```python
from build123d import *

# Parameters (mm, degrees)
F0_W     = 134.62
F0_H     = 76.2
F1_DEPTH = 15.875
F3_DEPTH = 76.201
F5_DEPTH = 83.5152


with BuildPart() as f1:
    # F0 (on Top) → F1 (new body, symmetric)
    with BuildSketch(Plane.XY):
        Rectangle(F0_W, F0_H)
    extrude(amount=F1_DEPTH, both=True)

    # F2 (on face) → F3 (cut, through all)
    with BuildSketch(Plane.XZ.offset(38.1)):
        Polygon((-33.401, 15.875), (-49.911, 15.875), (-49.911, 0), (-54.6735, 0), (-54.6735, -8.255), (-28.6385, -8.255), (-28.6385, 0), (-33.401, 0), align=None)
    extrude(amount=-F3_DEPTH, mode=Mode.SUBTRACT)

    # F4 (on face) → F5 (cut)
    with BuildSketch(Plane.YZ.offset(67.31)):
        with BuildLine():
            ThreePointArc((13.990774, -8.396005), (0.020774, 5.573995), (-13.949226, -8.396005))
            Line((-13.949226, -8.396005), (13.990774, -8.396005))
        make_face()
        Polygon((-13.949226, -8.396005), (-22.204226, -8.396005), (-17.886226, -15.875), (17.927774, -15.875), (22.245774, -8.396005), (13.990774, -8.396005), align=None)
    extrude(amount=-F5_DEPTH, mode=Mode.SUBTRACT)


with BuildPart() as f6_1:
    # F6: copy of F1
    add(f1.part)


solid = f1.part
```
Part model, mm, in its own coordinate system. A direction names the side the tool comes from. Give positions to 0.01 mm unless a question says otherwise; leave off trailing zeros. Order: outer loops, then holes, each group sorted by start corner. A loop starts at its lowest first (then second) coordinate and runs counter-clockwise, first axis right, second up. Notation, with made-up numbers: M 20,55 L 59,55 A30 cw 59,94 Z; hole C 27.25,6.5 d9. An arc over 180 degrees is marked long. Use a Markdown table: item, result. Add a question column.
(1) Drop flat-ended pins along their axis: P1, Ø9, axis at y = -5, z = -3.5, coming from the +X side; P2, Ø8, axis at x = -40, y = -17, coming from the +Z side (3 decimals). Give the stop position or say it passes through.
(2) Saw through at C-C, the plane x = -3.5. Give the cut face in (y, z) (3 decimals), and give its area (3 significant figures).
(3) Mould opens along Z. For faces 4 (the face through (26.14, 0.33, 5.57)), 5 (the face through (-59, 1, 15.875)), 6 (the face through (26.137, -20.075, -12.083)) say: +Z half, -Z half, draft (parallel to the pull), parting line (faces both ways), or undercut.
(4) Saw through at A-A, the plane z = -5. Give the cut face in (x, y).
(5) 3-axis set-ups, long thin cutter, end or side, ignore diameter. For faces 1 (the face through (-49.911, -1, 8)), 2 (the face through (26, -18, -8.396)), 3 (the face through (-54.674, -1, -4)): which of +Z, -Z, +X, -X, +Y, -Y reach the whole face in a straight line?
(6) Probe line 1 along X through (y, z) = (1, 7); line 2 along X through (y, z) = (-30.5, -7.5); line 3 along Z through (x, y) = (-29.5, -14.5) (3 decimals). List the from-to ranges inside material, lowest first. Write a range as [from, to].
(7) Saw through at B-B, the plane y = -26. Give the cut face in (x, z) (1 decimal), and give its area (3 significant figures).
(8) Saw through at D-D, the plane z = -14. Give the cut face in (x, y).
Answer key:
| question | item | result |
|---|---|---|
| 1 | P1 | x = -16.21 |
| 1 | P2 | z = -8.255 |
| 2 | outline | M -38.1,-15.875 L -17.886,-15.875 L -22.204,-8.396 L -13.949,-8.396 A13.97 cw 13.991,-8.396 L 22.246,-8.396 L 17.928,-15.875 L 38.1,-15.875 L 38.1,15.875 L -38.1,15.875 Z |
| 2 | area | 1,810 mm^2 |
| 3 | face 4 | -Z half |
| 3 | face 5 | +Z half |
| 3 | face 6 | undercut |
| 4 | outline | M -67.31,-38.1 L -54.67,-38.1 L -54.67,38.1 L -67.31,38.1 Z; M -28.64,-38.1 L 67.31,-38.1 L 67.31,-13.53 L -16.21,-13.53 L -16.21,13.57 L 67.31,13.57 L 67.31,38.1 L -28.64,38.1 Z |
| 5 | face 1 | +Z, +Y, -Y |
| 5 | face 2 | +X |
| 5 | face 3 | +Y, -Y |
| 6 | line 1 | [-67.31, -49.91], [-33.4, 67.31] |
| 6 | line 2 | [-67.31, -54.67], [-28.64, 67.31] |
| 6 | line 3 | [-15.875, -8.255], [0, 15.875] |
| 7 | outline | M -67.3,-15.9 L 67.3,-15.9 L 67.3,15.9 L -33.4,15.9 L -33.4,0 L -28.6,0 L -28.6,-8.3 L -54.7,-8.3 L -54.7,0 L -49.9,0 L -49.9,15.9 L -67.3,15.9 Z |
| 7 | area | 3,800 mm^2 |
| 8 | outline | M -67.31,-38.1 L 67.31,-38.1 L 67.31,-18.97 L -16.21,-18.97 L -16.21,19.01 L 67.31,19.01 L 67.31,38.1 L -67.31,38.1 Z |
